Can you work these out from the model? Positions are in its coordinate system, mm. Face numbers are marked on the shaded views. A direction names the side the tool comes from. Give positions to 0.01 mm unless a question says otherwise; leave off trailing zeros. Order: outer loops, then holes, each group sorted by start corner. A loop starts at its lowest first (then second) coordinate and runs counter-clockwise, first axis right, second up. Notation, with made-up numbers: (59, 6.5) - (111, 6.5) arc R20 cw to (111, 12.5) - close; hole circle Ø5 at (77, 74). An arc over 180 degrees is marked (long way). Answer as CSV lines item,"result".
```python
from build123d import *

# Parameters (mm, degrees)
F0_W          = 60
F0_H          = 60
F0_W_2        = 55
F0_H_2        = 55
F1_DEPTH      = 268.7
F3_DEPTH      = 75
F3_DEPTH_BACK = 75


with BuildPart() as f1:
    # F0 (on Front) → F1 (new body)
    with BuildSketch(Plane.XZ):
        Rectangle(F0_W, F0_H)
        Rectangle(F0_W_2, F0_H_2, mode=Mode.SUBTRACT)
    extrude(amount=-F1_DEPTH)

    # F2 (on face) → F3 (cut, two sides)
    with BuildSketch(Plane(origin=(-30, 0, 0), x_dir=(0, -1, 0), z_dir=(-1, 0, 0))) as f3_sk:
        Polygon((0, -30), (0, 30), (-60, -30), align=None)
        Polygon((-208.7, -30), (-268.7, 30), (-268.7, -30), align=None)
    extrude(amount=-F3_DEPTH, mode=Mode.SUBTRACT)
    extrude(f3_sk.sketch, amount=-F3_DEPTH_BACK, mode=Mode.SUBTRACT)


solid = f1.part
```
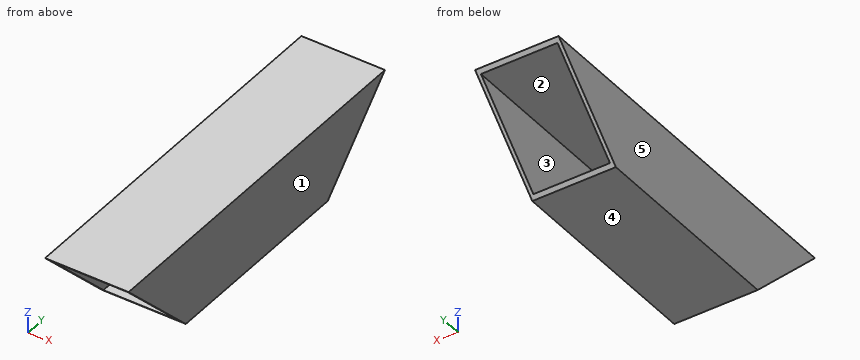
1) I want a section at A-A on x = -11. Write out the boundary of the cut face in (y, z), plus the area to 3 significant figures.
Answer block:
outline,"(0, 30) - (2.5, 27.5) - (266.2, 27.5) - (268.7, 30) - close; (57.5, -27.5) - (60, -30) - (208.7, -30) - (211.2, -27.5) - close"
area,"1,040 mm2"
2) I'm going to push a flat-ended pin straight in: P1, Ø2, axis at x = 20.5, y = 225.5, coming from the -Z side. Where does the tip first touch, or does it pass through?
Answer block:
P1,"z = 27.5"
3) I want a section at B-B on z = 16. Write out the boundary of the cut face in (x, y), plus the area to 3 significant figures.
Answer block:
outline,"(-30, 14) - (-27.5, 14) - (-27.5, 254.7) - (-30, 254.7) - close; (27.5, 14) - (30, 14) - (30, 254.7) - (27.5, 254.7) - close"
area,"1,200 mm2"
4) I want a section at C-C on y = 252.5. Write out the boundary of the cut face in (x, z), plus the area to 4 significant figures.
Answer block:
outline,"(-30, 13.8) - (-27.5, 13.8) - (-27.5, 27.5) - (27.5, 27.5) - (27.5, 13.8) - (30, 13.8) - (30, 30) - (-30, 30) - close"
area,"218.5 mm2"
5) If we mould it in two halves opening along X, with no side actions, what happens to the marked faces 3, 4 and 5? For each: +X half, -X half, draft (parallel to the pull), parting line (faces both ways), or undercut.
Answer block:
face 3,"undercut"
face 4,"draft"
face 5,"-X half"
6) Which directions (+Z, -Z, +X, -X, +Y, -Y) give clear straight access to the entire face, cutting with the end or side of a thin tool? Please do the marked faces 1 and 2.
Answer block:
face 1,"+Z, -Z, +X, +Y, -Y"
face 2,"+Y, -Y"
7) I want a section at D-D on y = 160. Write out the boundary of the cut face in (x, z), plus the area to 3 significant figures.
Answer block:
outline,"(-30, -30) - (30, -30) - (30, 30) - (-30, 30) - close; hole (-27.5, -27.5) - (27.5, -27.5) - (27.5, 27.5) - (-27.5, 27.5) - close"
area,"575 mm2"
8) I need wall thicknesses on line 1 along X through (y, z) = (101, 13); line 2 along Z through (x, y) = (-20.5, 239). Which ranges of each line are inside material? Lowest first, please. Write a range as [from, to].
Answer block:
line 1,"[-30, -27.5], [27.5, 30]"
line 2,"[27.5, 30]"
